Read the model definition and answer for the solid it produces. Units are mm, in the model's axes. A direction names the side the tool comes from. Coordinates: 2 decimals unless noted, no trailing zeros. Loops run counter-clockwise (first coordinate to the right, second up) from the corner with the lowest first, then second, coordinate; pieces in that order, holes last.
Autodesk Inventor part; units mm, degrees
ref_plane "YZ Plane" through (0, 0, 0) normal (1, 0, 0) x (0, 1, 0)
ref_plane "XZ Plane" through (0, 0, 0) normal (0, 1, 0) x (-1, 0, 0)
ref_plane "XY Plane" through (0, 0, 0) normal (0, 0, 1) x (1, 0, 0)
sketch "Sketch1" plane through (0, 0, 0) normal (1, 0, 0) x (0, 1, 0)
  circle A0 centre (0, 0) radius 1
  dimension "d0" = 2
sketch "Sketch2" plane through (0, 0, 0) normal (0, 1, 0) x (-1, 0, 0)
  line L0 (0, 0) -> (-3.5, 0)
  line L1 (-4, -0.5) -> (-4, -84.5)
  line L2 (-3.5, -85) -> (0, -85)
  arc A0 (-3.5, 0) -> (-4, -0.5) centre (-3.5, -0.5) ccw
  arc A1 (-4, -84.5) -> (-3.5, -85) centre (-3.5, -84.5) ccw
  point P0 (-4, 0)
  point P1 (-4, -85)
  dimension "d1" = 4
  dimension "d2" = 85
  dimension "d3" = 0.5
sweep "Sweep1" add profiles "Sketch1" path "Sketch2"
properties part number "Styrepind" material "Steel"
Q1. Determine the mould class of faces 1 (the face through (2, 0, -1)), 2 (the face through (0, 0, -85)) for opening direction Z: +Z half, -Z half, draft (parallel to the pull), parting line (faces both ways), or undercut.
Findings below:
face 1: undercut
face 2: draft
Q2. A cutting plane is placed at A-A (z = -56.5). Give the vertices of the cut face in (x, y), then the cut area to 3 significant figures.
Findings below:
outline: circle Ø2 at (4, 0)
area: 3.14 mm2
Q3. Which of the six approach directions +Z, -Z, +X, -X, +Y, -Y give full straight-line access (tool end or side, diameter ignored) to faces 3 (the face through (0, 0, 0)), 4 (the face through (5, 0, -43))?
Findings below:
face 3: +Z, -Z, -X, +Y, -Y
face 4: none
Q4. Straight lines are drawn through the part: probe 1 along Z at (x, y) = (1.5, 0.05); probe 2 along X at (y, z) = (0.15, -78); probe 3 along Z at (x, y) = (0.85, -0.65). For each, find the intervals that lie inside material, in ascending order.
Findings below:
probe 1: z = -86 to -84, -1 to 1
probe 2: x = 3.01 to 4.99
probe 3: z = -85.76 to -84.24, -0.76 to 0.76
Q5. A flat-ended cylindrical pin translates along its axis: pin 1 Ø1.5 at (x, z) = (3, -63.5) entering from -Y. Find the tip coordinate at first contact, or state that the pin passes through.
Findings below:
pin 1: stops at y = -0.97
